```python
from build123d import *

# Parameters (mm, degrees)
SKETCH1_W           = 3.175
SKETCH1_H           = 31.75
SKETCH1_W_2         = 28.575
SKETCH1_H_2         = 3.175
BOSS_EXTRUDE1_DEPTH = 50.8
POT_MOUNT_REACH     = 5.175
SKETCH2_R           = 3.683
BASE_MOUNT_REACH    = 5.175
SKETCH3_R           = 3.96875


with BuildPart() as part:
    # Sketch1 → Boss-Extrude1 (new body)
    with BuildSketch(Plane.XY):
        with Locations((1.5875, 15.875)):
            Rectangle(SKETCH1_W, SKETCH1_H)
        with Locations((17.4625, 1.5875)):
            Rectangle(SKETCH1_W_2, SKETCH1_H_2)
    extrude(amount=BOSS_EXTRUDE1_DEPTH)

    # Sketch2 → Pot Mount (cut, up to next)
    with BuildSketch(Plane(origin=(3.175, 0, 0), x_dir=(0, 0, -1), z_dir=(1, 0, 0)), mode=Mode.PRIVATE) as pot_mount_sk1:
        with Locations((-25.4, 19.05)):
            Circle(SKETCH2_R)
    pot_mount_tool1 = extrude(pot_mount_sk1.sketch, amount=-POT_MOUNT_REACH, mode=Mode.PRIVATE) & part.part
    add(pot_mount_tool1.solids().sort_by_distance((3.175, 19.05, 25.4))[0], mode=Mode.SUBTRACT)

    # Sketch3 → Base Mount (cut, up to next)
    with BuildSketch(Plane(origin=(0, 3.175, 0), x_dir=(1, 0, 0), z_dir=(0, 1, 0)), mode=Mode.PRIVATE) as base_mount_sk1:
        with Locations((22.225, -38.1)):
            Circle(SKETCH3_R)
    base_mount_tool1 = extrude(base_mount_sk1.sketch, amount=-BASE_MOUNT_REACH, mode=Mode.PRIVATE) & part.part
    add(base_mount_tool1.solids().sort_by_distance((22.225, 3.175, 38.1))[0], mode=Mode.SUBTRACT)
    # Sketch3 → Base Mount (cut, up to next)
    with BuildSketch(Plane(origin=(0, 3.175, 0), x_dir=(1, 0, 0), z_dir=(0, 1, 0)), mode=Mode.PRIVATE) as base_mount_sk2:
        with Locations((22.225, -12.7)):
            Circle(SKETCH3_R)
    base_mount_tool2 = extrude(base_mount_sk2.sketch, amount=-BASE_MOUNT_REACH, mode=Mode.PRIVATE) & part.part
    add(base_mount_tool2.solids().sort_by_distance((22.225, 3.175, 12.7))[0], mode=Mode.SUBTRACT)


solid = part.part
```
Build history of the part. All positions in model axes, mm. A direction names the side the tool comes from. Round coordinates to 2 decimals unless told otherwise and drop trailing zeros. Order: outer loops, then holes, each group sorted by start corner. A loop starts at its lowest first (then second) coordinate and runs counter-clockwise, first axis right, second up. Notation, with made-up numbers: (-36.75, 45.25) - (16.25, 45.25) arc R17 ccw to (16.25, 78.25) - close; hole circle Ø5 at (48, 28). An arc over 180 degrees is marked (long way). Use a Markdown table: item, result.
1) Saw through at B-B on z = 25.4. Write the cut outline in (x, y) (3 decimals).
Recorded:
| item | result |
|---|---|
| outline | (0, 0) - (31.75, 0) - (31.75, 3.175) - (3.175, 3.175) - (3.175, 15.367) - (0, 15.367) - close; (0, 22.733) - (3.175, 22.733) - (3.175, 31.75) - (0, 31.75) - close |
2) Wall check: L1, parallel to Z at x = 22, y = 1.5; L2, parallel to X at y = 1, z = 38; L3, parallel to Y at x = 1.7, z = 25.4. Give the ranges that are in metal, low to high.
Recorded:
| item | result |
|---|---|
| L1 | z = 0 to 8.74, 16.66 to 34.14, 42.06 to 50.8 |
| L2 | x = 0 to 18.26, 26.19 to 31.75 |
| L3 | y = 0 to 15.37, 22.73 to 31.75 |
3) Saw through at D-D on z = 38.1. Write the cut outline in (x, y) (3 decimals).
Recorded:
| item | result |
|---|---|
| outline | (0, 0) - (18.256, 0) - (18.256, 3.175) - (3.175, 3.175) - (3.175, 31.75) - (0, 31.75) - close; (26.194, 0) - (31.75, 0) - (31.75, 3.175) - (26.194, 3.175) - close |
4) Saw through at A-A on y = 19.05. Write the cut outline in (x, z) (3 decimals), and give its area (3 significant figures).
Recorded:
| item | result |
|---|---|
| outline | (0, 0) - (3.175, 0) - (3.175, 21.717) - (0, 21.717) - close; (0, 29.083) - (3.175, 29.083) - (3.175, 50.8) - (0, 50.8) - close |
| area | 138 mm² |
5) Flat gauge pins, fed straight in: pin 1 Ø8 at (y, z) = (27.5, 45) entering from +X (3 decimals); pin 2 Ø3 at (x, z) = (19, 11) entering from +Y (3 decimals). Where does each tip first touch, or does it go through?
Recorded:
| item | result |
|---|---|
| pin 1 | stops at x = 3.175 |
| pin 2 | stops at y = 3.175 |
6) Pull direction Z, two halves, no side cores. Call faces 1 (the face through (1.61, 17.639, 21.998)), 2 (the face through (9, 3, 50.8)), 3 (the face through (9, 3, 0)): pulls with the +Z half, pulls with the -Z half, needs draft (parallel to the pull), parting line crosses it, or undercut.
Recorded:
| item | result |
|---|---|
| face 1 | undercut |
| face 2 | pulls with the +Z half |
| face 3 | pulls with the -Z half |
7) Saw through at C-C on x = 20. Write the cut outline in (y, z) (3 decimals).
Recorded:
| item | result |
|---|---|
| outline | (0, 0) - (3.175, 0) - (3.175, 9.414) - (0, 9.414) - close; (0, 15.986) - (3.175, 15.986) - (3.175, 34.814) - (0, 34.814) - close; (0, 41.386) - (3.175, 41.386) - (3.175, 50.8) - (0, 50.8) - close |
8) Tool access for faces 4 (the face through (16, 0, 25)), 5 (the face through (3.175, 14, 25)): list every direction of +Z, -Z, +X, -X, +Y, -Y with a clear straight run to the whole face (end or side of a thin tool).
Recorded:
| item | result |
|---|---|
| face 4 | +Z, -Z, +X, -X, -Y |
| face 5 | +Z, -Z, +X, +Y |
